Check sheet for the drawn part. Datum: minimum x, y, z corner. Units: mm. A direction names the side the tool comes from. Give positions to 0.01 mm unless a question says otherwise; leave off trailing zeros. Loops run counter-clockwise (first coordinate to the right, second up) from the corner with the lowest first, then second, coordinate; pieces in that order, holes last.
1. Cross-section at D-D, the plane x = 27.5. Record the cut outline in (y, z), plus the area to 3 significant figures.
2. Material ranges on L1, parallel to Z at x = 15, y = 7.75; L2, parallel to Z at x = 2.5, y = 1.5; L3, parallel to X at y = 1.5, z = 27.5 (1 decimal), recorded low to high.
3. Cross-section at B-B, the plane z = 27.5. Record the cut outline in (x, y).
4. Release check for a two-part mould opening along X. For the marked faces 4, 5, 6 and 7 record: +X half, -X half, draft (parallel to the pull), parting line (faces both ways), or undercut.
5. Go/stop test with flat-tipped pins: pin 1 Ø3 at (y, z) = (9.5, 23.5) entering from +X; pin 2 Ø2.5 at (x, z) = (2, 18.5) entering from +Y; pin 3 Ø5 at (y, z) = (9, 21) entering from -X. Record where each tip stops, or that it passes through.
6. Cross-section at A-A, the plane x = 15. Record the cut outline in (y, z).
7. Tool access check on the marked faces 1, 2 and 3. Record the directions out of +Z, -Z, +X, -X, +Y, -Y that give a thin tool (end or side, any length) a straight path to the whole face; none if there is none.
8. Cross-section at C-C, the plane z = 10.75. Record the cut outline in (x, y).
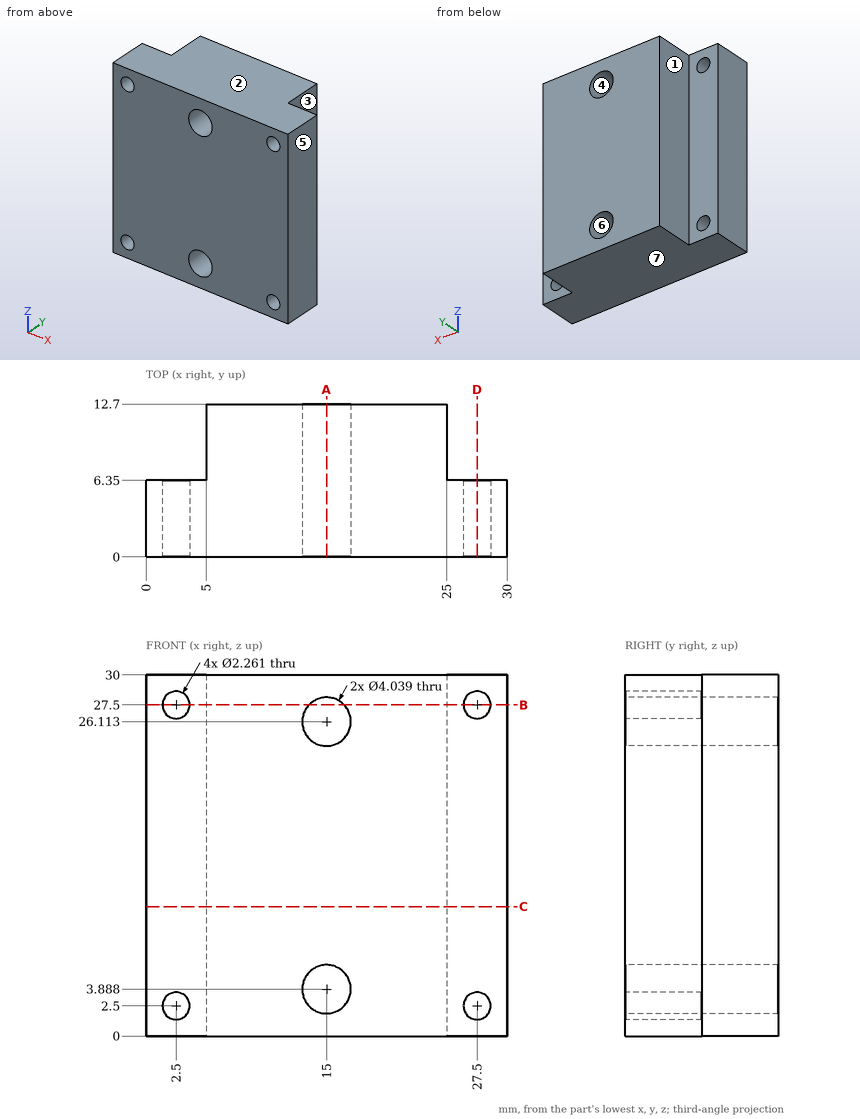
Result:
1. outline: (0, 0) - (6.35, 0) - (6.35, 1.37) - (0, 1.37) - close; (0, 3.63) - (6.35, 3.63) - (6.35, 26.37) - (0, 26.37) - close; (0, 28.63) - (6.35, 28.63) - (6.35, 30) - (0, 30) - close
1. area: 162 mm2
2. L1: z = 0 to 1.87, 5.91 to 24.09, 28.13 to 30
2. L2: z = 0 to 1.37, 3.63 to 26.37, 28.63 to 30
2. L3: x = 0 to 1.4, 3.6 to 13.5, 16.5 to 26.4, 28.6 to 30
3. outline: (0, 0) - (1.37, 0) - (1.37, 6.35) - (0, 6.35) - close; (3.63, 0) - (13.53, 0) - (13.53, 12.7) - (5, 12.7) - (5, 6.35) - (3.63, 6.35) - close; (16.47, 0) - (26.37, 0) - (26.37, 6.35) - (25, 6.35) - (25, 12.7) - (16.47, 12.7) - close; (28.63, 0) - (30, 0) - (30, 6.35) - (28.63, 6.35) - close
4. face 4: undercut
4. face 5: +X half
4. face 6: undercut
4. face 7: draft
5. pin 1: stops at x = 25
5. pin 2: stops at y = 6.35
5. pin 3: stops at x = 5
6. outline: (0, 0) - (12.7, 0) - (12.7, 1.87) - (0, 1.87) - close; (0, 5.91) - (12.7, 5.91) - (12.7, 24.09) - (0, 24.09) - close; (0, 28.13) - (12.7, 28.13) - (12.7, 30) - (0, 30) - close
7. face 1: +Z, -Z, -X, +Y
7. face 2: +Z, +X, -X, +Y, -Y
7. face 3: +Z, -Z, +X, +Y
8. outline: (0, 0) - (30, 0) - (30, 6.35) - (25, 6.35) - (25, 12.7) - (5, 12.7) - (5, 6.35) - (0, 6.35) - close
